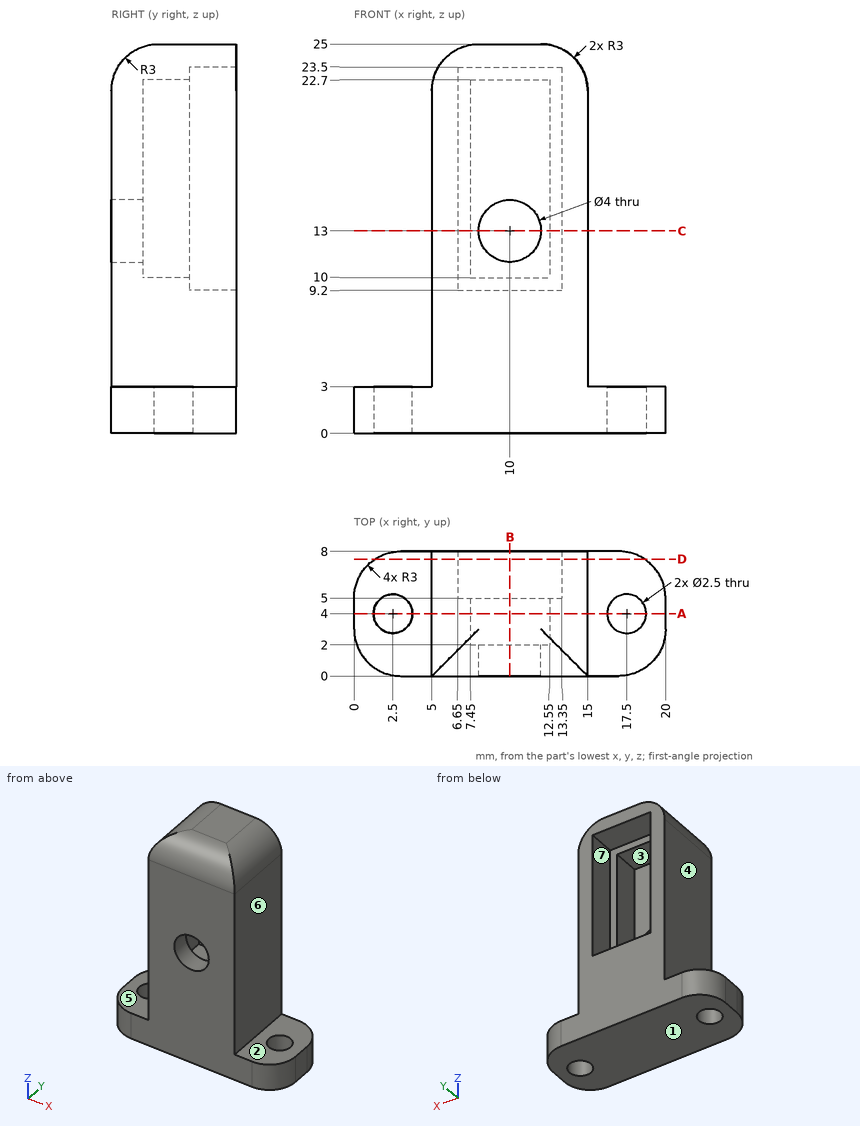
Source: three-view drawing plus pictorial views. Frame: mm from the lowest corner of the part. A direction names the side the tool comes from. Round coordinates to 2 decimals unless told otherwise and drop trailing zeros. Write each loop counter-clockwise with the first axis right and the second up, starting at its lowest first coordinate (ties: lowest second). Pieces come first, ordered by that corner, then holes. Notation, with made-up numbers: M -21,72.5 L 2,72.5 A24 ccw 2,82.5 Z; hole C 14,13.5 d4. An arc over 180 degrees is marked long. One line per item, written item: value. Start each with the question number.
Item 1: Section query A-A (y = 4). Return the cut outline in (x, z), plus the area to 3 significant figures.
Item 2: Section query C-C (z = 13). Return the cut outline in (x, y).
Item 3: Set-up query: the marked faces 1, 2, 3 and 4. Return all of +Z, -Z, +X, -X, +Y, -Y with unobstructed straight access to the full face (end or side cutting, diameter ignored); none if empty.
Item 4: Section query B-B (x = 10). Return the cut outline in (y, z), plus the area to 3 significant figures.
Item 5: Section query D-D (y = 7.5). Return the cut outline in (x, z), plus the area to 3 significant figures.
Item 6: Ray query, L1, parallel to X at y = 1.1, z = 13; L2, parallel to Z at x = 8.75, y = 3.5; L3, parallel to X at y = 3.75, z = 17. Return the intervals inside material, ascending. Write a range as from..to.
Item 7: Pin query (flat end, axial travel): pin 1 (2.5 mm diameter, centred on y = 4.5, z = 10, fed in from +X); pin 2 (2.5 mm diameter, centred on y = 3, z = 14, fed in from -X); pin 3 (1.5 mm diameter, centred on x = 3.5, y = 6, fed in from +Z). Return the tip coordinate at first contact, or that it passes through.
Item 8: Mould query, pull axis Z, two halves, no side actions, for the marked faces 5, 6 and 7. Classes: pulls with the +Z half, pulls with the -Z half, needs draft (parallel to the pull), parting line crosses it, or undercut.
Result set:
1. outline: M 0,0 L 1.25,0 L 1.25,3 L 0,3 Z; M 3.75,0 L 16.25,0 L 16.25,3 L 15,3 L 15,22 A3 ccw 12,25 L 8,25 A3 ccw 5,22 L 5,3 L 3.75,3 Z; M 18.75,0 L 20,0 L 20,3 L 18.75,3 Z; hole M 7.45,10 L 12.55,10 L 12.55,22.7 L 7.45,22.7 Z
1. area: 196 mm²
2. outline: M 5,0 L 8,0 L 8,2 L 7.45,2 L 7.45,5 L 6.65,5 L 6.65,8 L 5,8 Z; M 12,0 L 15,0 L 15,8 L 13.35,8 L 13.35,5 L 12.55,5 L 12.55,2 L 12,2 Z
3. face 1: -Z, +X, -X, +Y, -Y
3. face 2: +Z, +X, +Y, -Y
3. face 3: +Y
3. face 4: +Z, -X, +Y, -Y
4. outline: M 0,0 L 8,0 L 8,9.2 L 5,9.2 L 5,10 L 2,10 L 2,11 L 0,11 Z; M 0,15 L 2,15 L 2,22.7 L 5,22.7 L 5,23.5 L 8,23.5 L 8,25 L 3,25 A3 ccw 0,22 Z
4. area: 109 mm²
5. outline: M 1.34,0 L 18.66,0 L 18.66,3 L 15,3 L 15,22 A3 ccw 12,25 L 8,25 A3 ccw 5,22 L 5,3 L 1.34,3 Z; hole M 6.65,9.2 L 13.35,9.2 L 13.35,23.5 L 6.65,23.5 Z
5. area: 172 mm²
6. L1: x = 5..8, 12..15
6. L2: z = 0..10, 22.7..25
6. L3: x = 5..7.45, 12.55..15
7. pin 1: stops at x = 15
7. pin 2: stops at x = 5
7. pin 3: stops at z = 3
8. face 5: pulls with the +Z half
8. face 6: needs draft
8. face 7: undercut
